Read the model definition and answer for the solid it produces. Units are mm, in the model's axes. A direction names the side the tool comes from. Coordinates: 2 decimals unless noted, no trailing zeros. Write each loop counter-clockwise with the first axis right and the second up, starting at its lowest first coordinate (ties: lowest second). Pieces come first, ordered by that corner, then holes. Notation, with made-up numbers: (10, 35.5) -> (47, 35.5) arc R9 cw to (47, 45.5) -> close; hole circle Ø1 at (9.5, 51.25). An arc over 180 degrees is marked (long way). Answer as a JSON object with one key per item and string values. Group by question number.
(1) Flat-ended cylindrical pins translate along their axes: P1, Ø2, axis at x = -77, z = 11, coming from the -Y side; P2, Ø3, axis at x = -308, z = 7, coming from the -Y side. Find the tip coordinate at first contact, or state that the pin passes through.
(2) Find section D-D (y = -228). Give the vertices of the cut face in (x, z).
(3) Which of the six approach directions +Z, -Z, +X, -X, +Y, -Y give full straight-line access (tool end or side, diameter ignored) to faces 1 (the face through (-6, 81, 20)), 2 (the face through (-359.425, -172.828, 10.14))?
(4) Straight lines are drawn through the part: L1, parallel to Y at x = -32, z = 6.5; L2, parallel to X at y = -303, z = 5; L3, parallel to X at y = -262, z = 17.25. For each, find the intervals that lie inside material, in ascending order.
(5) Find section C-C (x = -203). Give the vertices of the cut face in (y, z), then the cut area to 3 significant figures.
(6) Find section B-B (z = 12.5). Give the vertices of the cut face in (x, y), then the cut area to 3 significant figures.
(7) Find section A-A (y = -77). Give the vertices of the cut face in (x, z), then the cut area to 3 significant figures.
from build123d import *

# Parameters (mm, degrees)
F0_W     = 910
F0_H     = 690
F1_DEPTH = 20
F2_W     = 340
F2_H     = 340
F3_DEPTH = 25
F4_R     = 20


with BuildPart() as f1:
    # F0 (on Top) → F1 (new body)
    with BuildSketch(Plane.XY):
        Rectangle(F0_W, F0_H)
    extrude(amount=F1_DEPTH)

    # F2 (on face) → F3 (cut)
    with BuildSketch(Plane.XY.offset(20)):
        with Locations((-145, -175)):
            Rectangle(F2_W, F2_H)
        Polygon((-405, -345), (-315, -345), (-315, -5), align=None)
        Polygon((25, -5), (25, -345), (85, -345), align=None)
    extrude(amount=-F3_DEPTH, mode=Mode.SUBTRACT)

    # F4
    f4_edges = [f1.edges().sort_by_distance(p)[0] for p in [
        (-315, -5, 10),
        (25, -5, 10),
        (455, -345, 10),
        (455, 345, 10),
        (-455, 345, 10),
        (-455, -345, 10),
        (-405, -345, 10),
        (85, -345, 10),
    ]]
    fillet(f4_edges, radius=F4_R)


solid = f1.part
Results below:
{
 "1": {"P1": "stops at y = -5", "P2": "stops at y = -7.62"},
 "2": {"outline": "(-455, 0) -> (-374.03, 0) -> (-374.03, 20) -> (-455, 20) -> close; (64.35, 0) -> (455, 0) -> (455, 20) -> (64.35, 20) -> close"},
 "3": {"face 1": "+Z, +X, -X, +Y, -Y", "face 2": "+Z, -Z, -Y"},
 "4": {"L1": "y = -5 to 345", "L2": "x = -455 to -393.88, 77.59 to 455", "L3": "x = -455 to -383.03, 70.35 to 455"},
 "5": {"outline": "(-5, 0) -> (345, 0) -> (345, 20) -> (-5, 20) -> close", "area": "7,000 mm2"},
 "6": {"outline": "(-455, -325) arc R20 ccw to (-435, -345) -> (-420.39, -345) arc R20 ccw to (-401.06, -330.12) -> (-318.94, -19.88) arc R20 cw to (-299.61, -5) -> (8.22, -5) arc R20 cw to (27.92, -21.52) -> (82.08, -328.48) arc R20 ccw to (101.78, -345) -> (435, -345) arc R20 ccw to (455, -325) -> (455, 325) arc R20 ccw to (435, 345) -> (-435, 345) arc R20 ccw to (-455, 325) -> close", "area": "486,000 mm2"},
 "7": {"outline": "(-455, 0) -> (-334.06, 0) -> (-334.06, 20) -> (-455, 20) -> close; (37.71, 0) -> (455, 0) -> (455, 20) -> (37.71, 20) -> close", "area": "10,800 mm2"}
}
